```python
from build123d import *

# Parameters (mm, degrees)
SALIENTE_EXTRUIR1_DEPTH = 150.6
CROQUIS2_R              = 1.85
SALIENTE_EXTRUIR2_DEPTH = 70


with BuildPart() as part:
    # Croquis1 → Saliente-Extruir1 (new body)
    with BuildSketch(Plane.XY):
        with BuildLine():
            Line((-78.077598734, 121.298692457), (-78.077598734, 121.898692457))
            Line((-78.077598734, 121.898692457), (-77.177598734, 121.898692457))
            Line((-77.177598734, 121.898692457), (-77.177598734, 121.298692457))
            ThreePointArc((-77.177598734, 121.298692457), (-77.627598734, 116.339525931), (-78.077598734, 121.298692457))
        make_face()
    extrude(amount=SALIENTE_EXTRUIR1_DEPTH)

    # Croquis2 → Saliente-Extruir2 (add)
    with BuildSketch(Plane.XY.offset(150.6)):
        with Locations((-77.627598734, 118.839525931)):
            Circle(CROQUIS2_R)
    extrude(amount=SALIENTE_EXTRUIR2_DEPTH)


solid = part.part
```
Geometry check sheet. Reference: the model listing, model coordinates, mm. A direction names the side the tool comes from. Round coordinates to 2 decimals unless told otherwise and drop trailing zeros. Order: outer loops, then holes, each group sorted by start corner. A loop starts at its lowest first (then second) coordinate and runs counter-clockwise, first axis right, second up. Notation, with made-up numbers: (50, -13) - (108, -13) arc R14 ccw to (108, -5) - close; hole circle Ø8 at (33.25, 66.25). An arc over 180 degrees is marked (long way). Use a Markdown table: item, result. Add a question column.
1) Section check B-B (z = 179.5). Record the cut outline in (x, y).
2) Section check A-A (z = 146.5). Record the cut outline in (x, y), then the cut area to 3 significant figures.
3) Thickness scan on line 1 along Y through (x, z) = (-77.8, 55); line 2 along Y through (x, z) = (-78, 140.5); line 3 along Z through (x, y) = (-79, 117.5). Record the ranges inside material, lowest first.
4) Set-up check for faces 1 (the flat face through (-78, 119, 0)), 2 (the cylindrical face through (-76.633, 120.399, 185.11)): record each of +Z, -Z, +X, -X, +Y, -Y from which the full face is reachable in a straight line by a thin tool's end or side.
5) Gauge pin test, flat ends, axial feed: P1, Ø2, axis at x = -79, y = 117, coming from the +Z side; P2, Ø3, axis at y = 121, z = 194, coming from the +X side; P3, Ø3, axis at x = -78.5, z = 167, coming from the +Y side. Record the tip position at first contact, or that the pin passes through.
Established:
| question | item | result |
|---|---|---|
| 1 | outline | circle Ø3.7 at (-77.63, 118.84) |
| 2 | outline | (-78.08, 121.3) arc R2.5 ccw (long way) to (-77.18, 121.3) - (-77.18, 121.9) - (-78.08, 121.9) - close |
| 2 | area | 20.2 mm2 |
| 3 | line 1 | 116.35 to 121.9 |
| 3 | line 2 | 116.37 to 121.9 |
| 3 | line 3 | 0 to 150.6 |
| 4 | face 1 | -Z, +X, -X, +Y, -Y |
| 4 | face 2 | +Z |
| 5 | P1 | z = 220.6 |
| 5 | P2 | x = -75.9 |
| 5 | P3 | y = 120.69 |
